from build123d import *

# Parameters (mm, degrees)
F1_DEPTH    = 3.3
F2_R        = 0.5
F3_T        = 0.5
F3_T3_DEPTH = 4.3
F5_DEPTH    = 0.5
F6_DEPTH    = 0.5


# Not quite as in the source:
# - a shell that OpenCascade refuses in one call is made with other operations: the cavity is built on its own and cut out


with BuildPart() as f1:
    # F0 (on Front) → F1 (new body)
    with BuildSketch(Plane.XZ):
        Polygon((-0.7, -2.4), (0, -2.4), (0.7, -2.4), (0.35, -4.4), (1.85, -4.4), (2.4, 1), (0, 1), (-2.4, 1), (-1.85, -4.4), (-0.35, -4.4), align=None)
    extrude(amount=F1_DEPTH)

    # F2
    f2_edges = [f1.edges().sort_by_distance(p)[0] for p in [
        (2.4, -1.65, 1),
        (1.85, -1.65, -4.4),
        (-0.35, -1.65, -4.4),
        (-2.4, -1.65, 1),
        (0.35, -1.65, -4.4),
        (-1.85, -1.65, -4.4),
    ]]
    fillet(f2_edges, radius=F2_R)

    # F3: shell of thickness 0.5, made by hand


with BuildPart() as f3_core1:
    # F3_t2: copy of F1
    add(f1.part)

    # the walls: a layer under each face that stays
    f3_faces = [f3_core1.faces().sort_by_distance(p)[0] for p in [
        (0.5762916395, -1.65, -3.1069049171),
        (0, -1.65, -2.4),
        (1.17171884, -1.65, -4.4),
        (-0.5762916395, -1.65, -3.1069049171),
        (2.1198397965, -1.65, -1.7506638158),
        (-1.17171884, -1.65, -4.4),
        (0, -1.65, 1),
        (-2.1198397965, -1.65, -1.7506638158),
    ]]
    thicken(f3_faces, amount=-F3_T, mode=Mode.SUBTRACT)

    # F3_s4 → F3_t3 (cut)
    with BuildSketch(Plane.XZ.offset(-0.5)):
        Polygon((0.6950748477, -2.4041380983), (1.1925152336, -2.4861901659), (1.2950985126, -1.9), (0.7, -1.9), align=None)
        Polygon((-0.6950748477, -2.4041380983), (-0.7, -1.9), (-1.2950985126, -1.9), (-1.1925152336, -2.4861901659), align=None)
    extrude(amount=F3_T3_DEPTH, mode=Mode.SUBTRACT)


with BuildPart() as f1_1:
    add(f1.part)

    # what is left inside the walls is the cavity
    f3_cavity = [f3_core1.part.solids().sort_by_distance(p)[0] for p in [
        (-1.617439, -2.2, -1.699493),
    ]]
    add(f3_cavity, mode=Mode.SUBTRACT)

    # F4 (on face) → F5 (join, through all)
    with BuildSketch(Plane.XY.offset(1)):
        Polygon((1.8464873155, -3.3), (-1.8464873155, -3.3), (0, -4.3), align=None)
    extrude(amount=-F5_DEPTH)

    # F4 (on face) → F6 (cut, through all)
    with BuildSketch(Plane.XY.offset(1)):
        Polygon((1.8464873155, 0), (-1.8464873155, 0), (0, -1), align=None)
    extrude(amount=-F6_DEPTH, mode=Mode.SUBTRACT)


solid = f1_1.part
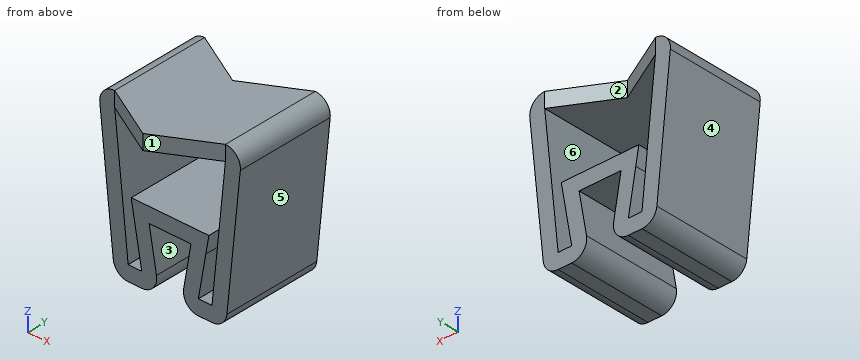
CAD build for the part. Positions are in the model's coordinates, mm. Face numbers are marked on the shaded views. A direction names the side the tool comes from. Give positions to 0.01 mm unless a question says otherwise; leave off trailing zeros. Order: outer loops, then holes, each group sorted by start corner. A loop starts at its lowest first (then second) coordinate and runs counter-clockwise, first axis right, second up. Notation, with made-up numbers: (25.5, -25.5) - (63.5, -25.5) arc R11 ccw to (63.5, -10.5) - close; hole circle Ø2 at (-3.75, 72.25). An arc over 180 degrees is marked (long way). Answer in a Markdown table with one row per item.
1. Tool access for the marked faces 1, 2 and 3: list every direction of +Z, -Z, +X, -X, +Y, -Y with a clear straight run to the whole face (end or side of a thin tool).
Data:
| item | result |
|---|---|
| face 1 | +Z, -Z, +X, -Y |
| face 2 | +Z, +Y |
| face 3 | +Y, -Y |
2. Probe probe 1 along Z at (x, y) = (-0.25, -1.6); probe 2 along X at (y, z) = (-1.05, -3.2); probe 3 along Y at (x, z) = (-1.9, -0.55). List the from-to ranges inside material, lowest first. Write a range as [from, to].
Data:
| item | result |
|---|---|
| probe 1 | z = [-2.4, -1.9], [0.5, 1] |
| probe 2 | x = [-1.97, -1.47], [-1.07, -0.56], [0.56, 1.07], [1.47, 1.97] |
| probe 3 | y = [-3.3, 0] |
3. Saw through at B-B, the plane z = -1.65. Give the cut face in (x, y).
Data:
| item | result |
|---|---|
| outline | (-2.13, -3.3) - (-1.63, -3.3) - (-1.63, 0) - (-2.13, 0) - close; (1.63, -3.3) - (2.13, -3.3) - (2.13, 0) - (1.63, 0) - close |
4. Saw through at C-C, the plane x = 1.6. Give the cut face in (y, z), plus the area to 3 significant figures.
Data:
| item | result |
|---|---|
| outline | (-3.43, 0.5) - (-0.13, 0.5) - (-0.13, 1) - (-3.43, 1) - close; (-3.3, -4.36) - (0, -4.36) - (0, -1.92) - (-3.3, -1.92) - close |
| area | 9.69 mm² |
5. Pull direction X, two halves, no side cores. Call the marked faces 4, 5 and 6: pulls with the +X half, pulls with the -X half, needs draft (parallel to the pull), parting line crosses it, or undercut.
Data:
| item | result |
|---|---|
| face 4 | pulls with the -X half |
| face 5 | pulls with the +X half |
| face 6 | undercut |
6. Flat gauge pins, fed straight in: pin 1 (1.5 mm diameter, centred on y = -3.5, z = -4, fed in from -X); pin 2 (0.7 mm diameter, centred on x = -0.5, y = -2, fed in from -Z). Where does each tip first touch, or does it go through?
Data:
| item | result |
|---|---|
| pin 1 | stops at x = -1.96 |
| pin 2 | stops at z = -4.39 |
7. Saw through at D-D, the plane x = -1.05. Give the cut face in (y, z).
Data:
| item | result |
|---|---|
| outline | (-3.73, 0.5) - (-0.43, 0.5) - (-0.43, 1) - (-3.73, 1) - close; (-3.3, -4.4) - (0, -4.4) - (0, -3.9) - (-3.3, -3.9) - close; (-3.3, -3.3) - (0, -3.3) - (0, -1.9) - (-3.3, -1.9) - close |
8. Saw through at A-A, the plane y = -2.25. Give the cut face in (x, z).
Data:
| item | result |
|---|---|
| outline | (-2.34, 0.45) - (-1.9, -3.95) arc R0.5 ccw to (-1.4, -4.4) - (-0.95, -4.4) arc R0.5 ccw to (-0.45, -3.81) - (-0.7, -2.4) - (0.7, -2.4) - (0.45, -3.81) arc R0.5 ccw to (0.95, -4.4) - (1.4, -4.4) arc R0.5 ccw to (1.9, -3.95) - (2.34, 0.45) arc R0.5 ccw to (1.85, 1) - (-1.85, 1) arc R0.5 ccw to start; hole (-1.85, 0.5) - (-1.4, -3.9) - (-0.95, -3.9) - (-1.3, -1.9) - (1.3, -1.9) - (0.95, -3.9) - (1.4, -3.9) - (1.85, 0.5) - close |
